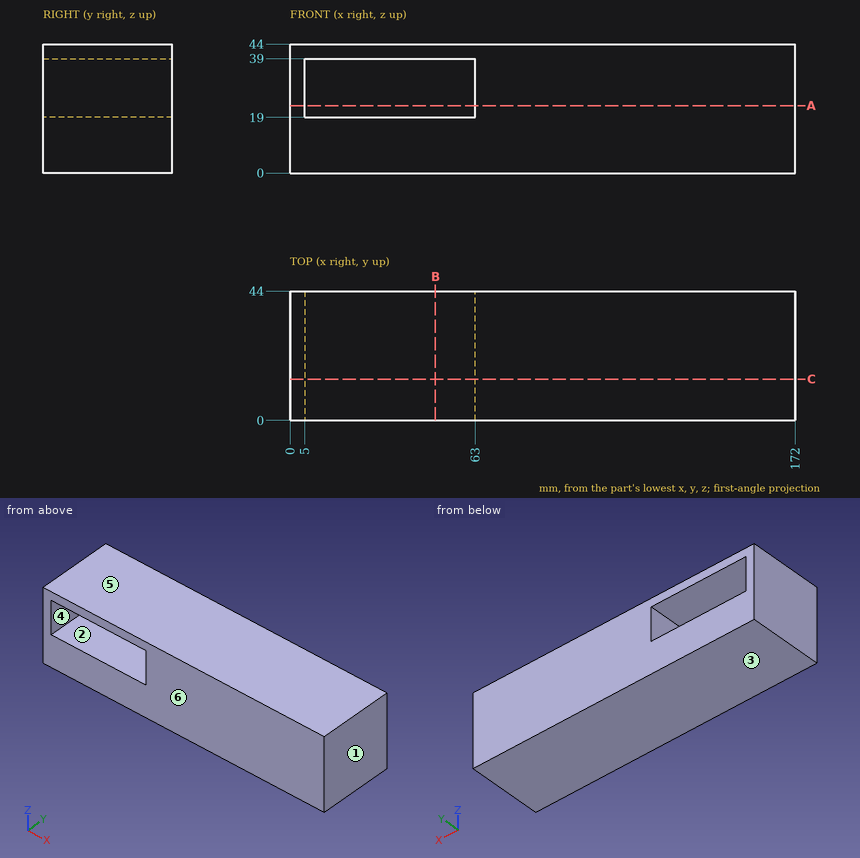
The drawing under review shows one solid part. Ordinate dimensions are in mm from its lowest x, y, z. A direction names the side the tool comes from. Give positions to 0.01 mm unless a question says otherwise; leave off trailing zeros. Order: outer loops, then holes, each group sorted by start corner. A loop starts at its lowest first (then second) coordinate and runs counter-clockwise, first axis right, second up. Notation, with made-up numbers: (36, 87) - (80, 87) arc R15 ccw to (80, 92) - close; hole circle Ø9 at (86.5, 12.25). An arc over 180 degrees is marked (long way). Answer as a JSON object with one key per item and string values. Group by question number.
Item 1: Machinability: for the marked faces 1 and 2, which of the approach directions +Z, -Z, +X, -X, +Y, -Y give a long, thin tool a straight path to every point of the face, cutting with its end or side? Answer none if there is none.
Item 2: Take a section at B-B on x = 49.5. Give the boundary of the cut face in (y, z).
Item 3: Clearance check with a flat-ended pin moving along its axis: pin 1 Ø5 at (x, z) = (46, 23.5) entering from +Y. State where the tip first meets the part, or that it passes through.
Item 4: Take a section at C-C on y = 14. Give the boundary of the cut face in (x, z).
Item 5: Take a section at A-A on z = 23. Give the boundary of the cut face in (x, y), and give its area (3 significant figures).
Item 6: Wall thickness on line 1 along Z through (x, y) = (51, 22); line 2 along X through (y, z) = (5.5, 31.5): over which ranges is each line inside the solid? List them lowest first.
Item 7: Draft analysis for pull direction Z (two halves, no side actions). For the marked faces 3, 4, 5 and 6, state which applies: pulls with the +Z half, pulls with the -Z half, needs draft (parallel to the pull), parting line crosses it, or undercut.
Reported:
{
 "1": {"face 1": "+Z, -Z, +X, +Y, -Y", "face 2": "+Y, -Y"},
 "2": {"outline": "(0, 0) - (44, 0) - (44, 19) - (0, 19) - close; (0, 39) - (44, 39) - (44, 44) - (0, 44) - close"},
 "3": {"pin 1": "through"},
 "4": {"outline": "(0, 0) - (172, 0) - (172, 44) - (0, 44) - close; hole (5, 19) - (63, 19) - (63, 39) - (5, 39) - close"},
 "5": {"outline": "(0, 0) - (5, 0) - (5, 44) - (0, 44) - close; (63, 0) - (172, 0) - (172, 44) - (63, 44) - close", "area": "5,020 mm^2"},
 "6": {"line 1": "0 to 19, 39 to 44", "line 2": "0 to 5, 63 to 172"},
 "7": {"face 3": "pulls with the -Z half", "face 4": "undercut", "face 5": "pulls with the +Z half", "face 6": "needs draft"}
}
